The model under review builds one solid part; all positions refer to its coordinate system, in mm. Coordinates: 2 decimals unless noted, no trailing zeros. Loops run counter-clockwise (first coordinate to the right, second up) from the corner with the lowest first, then second, coordinate; pieces in that order, holes last. Notation, with made-up numbers: (8.25, 42.25) - (57.25, 42.25) arc R7 cw to (57.25, 49.25) - close; hole circle Ø3 at (40, 57.5). An arc over 180 degrees is marked (long way). One line per item, written item: value. Start each with the question number.
1. We need section C-C, the plane z = 1.45. Give the boundary of the cut face in (x, y), then the cut area to 3 significant figures.
2. Mouldability with a two-part tool opening along Y and no side actions: class faces 1 (the face through (0, -9.75, 1)), 2 (the face through (0, 0, 0)), 3 (the face through (0, 0, 2)) as +Y half, -Y half, draft (parallel to the pull), parting line (faces both ways), or undercut.
3. Insertion check: P1, Ø3, axis at x = 1, y = -5, coming from the -Z side; P2, Ø1.9, axis at x = 0, y = 7, coming from the +Z side. Each pin has a flat end and moves straight along its axis. Give the tip position at first contact, or say it passes through.
4. We need section A-A, the plane x = 0. Count the separate pieces of the cut face and the enclosed holes in it, then the cut area to 3 significant figures.
5. To check wall thickness, follow line 1 (Y direction, x = 0, z = 1.85); line 2 (Y direction, x = 2.2, z = 2.1); line 3 (Y direction, x = -1.5, z = 0.4). State the ranges of each line that lie inside material, in increasing order.
6. We need section D-D, the plane z = 0.6. Give the boundary of the cut face in (x, y), then the cut area to 3 significant figures.
from build123d import *

# Parameters (mm, degrees)
SKETCH1_W             = 5.5
SKETCH1_H             = 5.5
SKETCH1_R             = 1.6
BOSS_EXTRUDE1_DEPTH   = 2.5
BOSS_EXTRUDE1_2_DEPTH = 2.5
SKETCH1_4_W           = 8.5
SKETCH1_4_H           = 2.75
BOSS_EXTRUDE2_DEPTH   = 2
CHAMFER1_SIZE         = 1.15


with BuildPart() as part:
    # Sketch1 → Boss-Extrude1 (new body)
    with BuildSketch(Plane(origin=(0, 0, 0), x_dir=(0, 1, 0), z_dir=(0, 0, 1))):
        with Locations((-7, 0)):
            Rectangle(SKETCH1_W, SKETCH1_H)
        with Locations(Location((-7, 0, 0), (0, 0, 270))):
            Circle(SKETCH1_R, mode=Mode.SUBTRACT)
    extrude(amount=BOSS_EXTRUDE1_DEPTH)



with BuildPart() as body_2:
    # Sketch1 → Boss-Extrude1 2 (new body)
    with BuildSketch(Plane(origin=(0, 0, 0), x_dir=(0, 1, 0), z_dir=(0, 0, 1))):
        with Locations((7, 0)):
            Rectangle(SKETCH1_W, SKETCH1_H)
        with Locations(Location((7, 0, 0), (0, 0, 270))):
            Circle(SKETCH1_R, mode=Mode.SUBTRACT)
    extrude(amount=BOSS_EXTRUDE1_2_DEPTH)


with BuildPart() as part_1:
    add(part.part)

    add(body_2.part)  # Boss-Extrude2 merges body 2
    # Sketch1<4> → Boss-Extrude2 (add)
    with BuildSketch(Plane(origin=(0, 0, 0), x_dir=(0, 1, 0), z_dir=(0, 0, 1))):
        with Locations((0, -1.375)):
            Rectangle(SKETCH1_4_W, SKETCH1_4_H)
        with Locations((0, 1.375)):
            Rectangle(SKETCH1_4_W, SKETCH1_4_H)
    extrude(amount=BOSS_EXTRUDE2_DEPTH)

    # Chamfer1
    chamfer1_edges = [part_1.edges().sort_by_distance(p)[0] for p in [
        (-1.6, 7, 0),
        (-1.6, -7, 0),
    ]]
    chamfer(chamfer1_edges, length=CHAMFER1_SIZE - 0.0001)  # a hair under: the kernel refuses the full size


solid = part_1.part
Findings below:
1. outline: (-2.75, -9.75) - (2.75, -9.75) - (2.75, 9.75) - (-2.75, 9.75) - close; hole circle Ø3.2 at (0, -7); hole circle Ø3.2 at (0, 7)
1. area: 91.2 mm2
2. face 1: -Y half
2. face 2: draft
2. face 3: undercut
3. P1: z = 0
3. P2: through
4. separate pieces: 3
4. enclosed holes: 0
4. area: 25.9 mm2
5. line 1: -9.75 to -8.6, -5.4 to 5.4, 8.6 to 9.75
5. line 2: -9.75 to -4.25, 4.25 to 9.75
5. line 3: -9.75 to -8.81, -5.19 to 5.19, 8.81 to 9.75
6. outline: (-2.75, -9.75) - (2.75, -9.75) - (2.75, 9.75) - (-2.75, 9.75) - close; hole circle Ø4.3 at (0, -7); hole circle Ø4.3 at (0, 7)
6. area: 78.2 mm2
